Here's how the part is built. I have some questions about the finished solid (model axes, mm). Face numbers are marked on the shaded views. A direction names the side the tool comes from. Round coordinates to 2 decimals unless told otherwise and drop trailing zeros. Write each loop counter-clockwise with the first axis right and the second up, starting at its lowest first coordinate (ties: lowest second). Pieces come first, ordered by that corner, then holes. Notation, with made-up numbers: M 88.25,60.25 L 98.25,60.25 A18 cw 98.25,72.25 Z; hole C 48.25,57.25 d7. An arc over 180 degrees is marked long. Use one line per item in the form item = value. Start each with the question number.
Q1. I want a section at D-D on x = -8. List the corners of the cut face in (y, z) for me.
Q2. I need wall thicknesses on line 1 along Y through (x, z) = (-8, 12.7); line 2 along X through (y, z) = (46, 13.2); line 3 along Y through (x, z) = (-84, 13.4). Which ranges of each line are inside material? Lowest first, please. Write a range as from..to.
Q3. I'm going to push flat-ended pins straight in: pin 1 Ø6 at (x, z) = (-27.5, 2) entering from +Y; pin 2 Ø3 at (x, z) = (-44, 7.5) entering from +Y. Where does each tip first touch, or does it pass through?
Q4. For the marked faces 1 and 2, which set-ups out of +Z, -Z, +X, -X, +Y, -Y let a thin tool reach every point of the face, with its end or its side?
Q5. I want a section at B-B on z = 9. List the corners of the cut face in (x, y) for me.
Q6. I want a section at C-C on y = 13.5. List the corners of the cut face in (x, z) for me.
Q7. I want a section at A-A on x = -84. List the corners of the cut face in (y, z) for me.
Q8. We'd pull the mould along Z, two halves only. Please class the marked faces 3, 4 and 5: +Z half, -Z half, draft (parallel to the pull), parting line (faces both ways), or undercut.
```python
from build123d import *

# Parameters (mm, degrees)
CROQUIS1_W              = 92
CROQUIS1_H              = 54
CROQUIS1_R              = 2
CROQUIS1_W_2            = 70
CROQUIS1_H_2            = 31.6
SALIENTE_EXTRUIR1_DEPTH = 14
CORTAR_EXTRUIR1_DEPTH   = 90
CROQUIS3_W              = 2
CROQUIS3_H              = 17.046925302
CORTAR_EXTRUIR2_DEPTH   = 12
CROQUIS4_W              = 8
CROQUIS4_H              = 13
CORTAR_EXTRUIR3_DEPTH   = 2
REDONDEO1_R             = 3
REDONDEO2_R             = 3
REDONDEO3_R             = 3


with BuildPart() as part:
    # Croquis1 → Saliente-Extruir1 (new body)
    with BuildSketch(Plane.XY):
        with Locations((-46, 27)):
            Rectangle(CROQUIS1_W, CROQUIS1_H)
        with Locations((-84, 46)):
            Circle(CROQUIS1_R, mode=Mode.SUBTRACT)
        with Locations((-8, 46)):
            Circle(CROQUIS1_R, mode=Mode.SUBTRACT)
        with Locations((-41, 18.4)):
            Rectangle(CROQUIS1_W_2, CROQUIS1_H_2, mode=Mode.SUBTRACT)
    extrude(amount=SALIENTE_EXTRUIR1_DEPTH)

    # Croquis2 → Cortar-Extruir1 (cut)
    with BuildSketch(Plane(origin=(0, 0, 0), x_dir=(0, 0, -1), z_dir=(1, 0, 0))):
        Polygon((-2, 36.953074698), (-2, 2), (-12, 2), (-12, 36.953074698), (-12, 54), (-2, 54), (0, 54), (0, 36.953074698), align=None)
    extrude(amount=-CORTAR_EXTRUIR1_DEPTH, mode=Mode.SUBTRACT)

    # Croquis3 → Cortar-Extruir2 (cut)
    with BuildSketch(Plane(origin=(0, 0, 0), x_dir=(-1, 0, 0), z_dir=(0, 0, -1))):
        with Locations((91, 45.476537349)):
            Rectangle(CROQUIS3_W, CROQUIS3_H)
    extrude(amount=-CORTAR_EXTRUIR2_DEPTH, mode=Mode.SUBTRACT)

    # Croquis4 → Cortar-Extruir3 (cut)
    with BuildSketch(Plane.ZY.offset(92)):
        with Locations((7, 8.840884816)):
            Rectangle(CROQUIS4_W, CROQUIS4_H)
    extrude(amount=-CORTAR_EXTRUIR3_DEPTH, mode=Mode.SUBTRACT)

    # Redondeo1
    redondeo1_edges = [part.edges().sort_by_distance(p)[0] for p in [
        (-92, 54, 13),
    ]]
    fillet(redondeo1_edges, radius=REDONDEO1_R)

    # Redondeo2
    redondeo2_edges = [part.edges().sort_by_distance(p)[0] for p in [
        (0, 54, 13),
    ]]
    fillet(redondeo2_edges, radius=REDONDEO2_R)

    # Redondeo3
    redondeo3_edges = [part.edges().sort_by_distance(p)[0] for p in [
        (0, 36.953074698, 1),
    ]]
    fillet(redondeo3_edges, radius=REDONDEO3_R)


solid = part.part
```
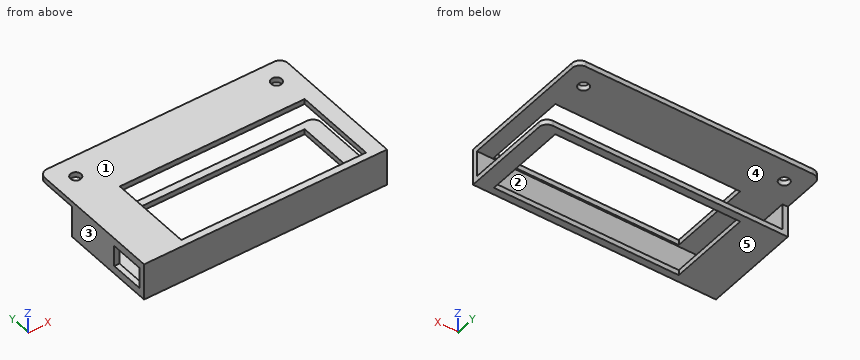
Reported:
q1.outline = M 0,0 L 2.6,0 L 2.6,2 L 2,2 L 2,12 L 2.6,12 L 2.6,14 L 0,14 Z; M 34.2,0 L 36.95,0 L 36.95,2 L 34.2,2 Z; M 34.2,12 L 44,12 L 44,14 L 34.2,14 Z; M 48,12 L 54,12 L 54,14 L 48,14 Z
q2.line_1 = 0..2.6, 34.2..44, 48..54
q2.line_2 = -92..-86, -82..-10, -6..0
q2.line_3 = 0..44, 48..54
q3.pin_1 = 36.95
q3.pin_2 = 2
q4.face_1 = +Z, +X, -X, +Y, -Y
q4.face_2 = +X, +Y
q5.outline = M -92,0 L 0,0 L 0,2 L -90,2 L -90,2.34 L -92,2.34 Z; M -92,15.34 L -90,15.34 L -90,36.95 L -92,36.95 Z
q6.outline = M -92,0 L -76,0 L -76,2 L -90,2 L -90,3 L -92,3 Z; M -92,11 L -90,11 L -90,12 L -76,12 L -76,14 L -92,14 Z; M -6,0 L 0,0 L 0,2 L -6,2 Z; M -6,12 L 0,12 L 0,14 L -6,14 Z
q7.outline = M 0,0 L 36.95,0 L 36.95,2 L 2,2 L 2,12 L 44,12 L 44,14 L 0,14 Z; M 48,12 L 54,12 L 54,14 L 48,14 Z
q8.face_3 = draft
q8.face_4 = undercut
q8.face_5 = -Z half
